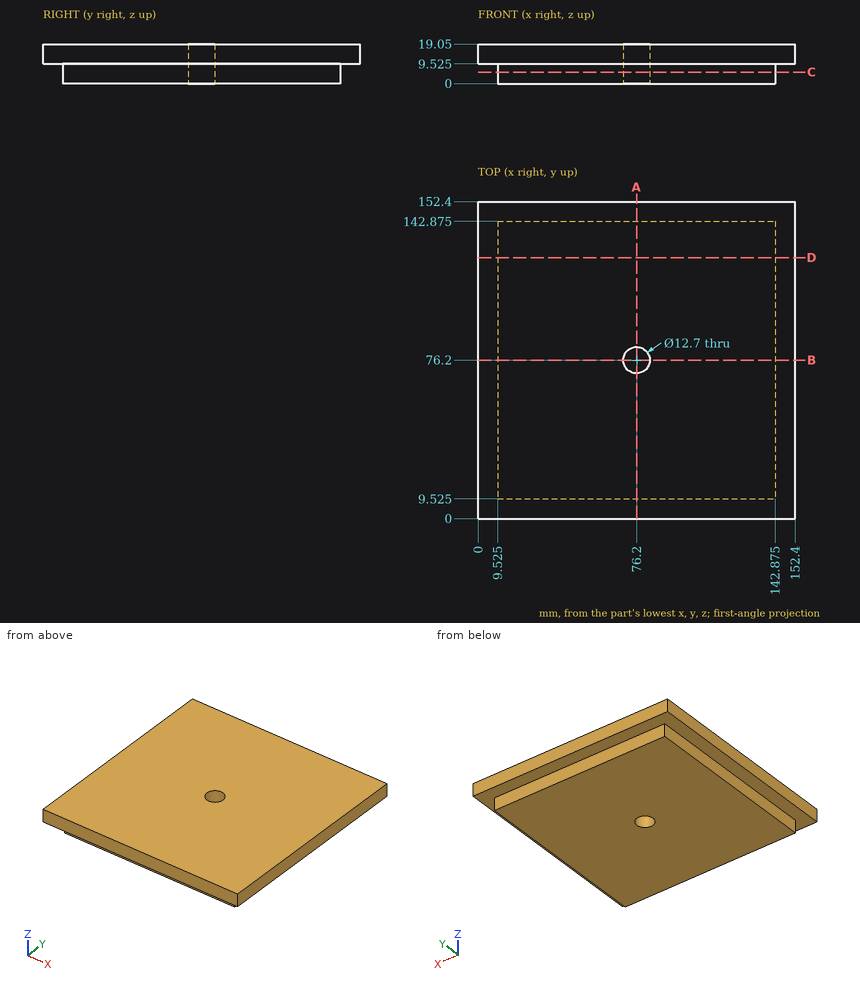
Design review of the part shown in the three views and the two pictorial views. Dimensions are in mm from the part's minimum x, y and z. Round coordinates to 2 decimals unless told otherwise and drop trailing zeros. Loops run counter-clockwise (first coordinate to the right, second up) from the corner with the lowest first, then second, coordinate; pieces in that order, holes last. Notation, with made-up numbers: M -1.75,-0.5 L 43.25,-0.5 A4 ccw 43.25,6.5 Z; hole C 8,50 d10. An arc over 180 degrees is marked long. Write item = value, one per line.
Item 1: Take a section at C-C on z = 5.5. Write out the cut boundary in (x, y) (3 decimals).
Return value:
outline = M 9.525,9.525 L 142.875,9.525 L 142.875,142.875 L 9.525,142.875 Z; hole C 76.2,76.2 d12.7
Item 2: Take a section at D-D on y = 125.5. Write out the cut boundary in (x, z) (3 decimals), then the cut area to 3 significant figures.
Return value:
outline = M 0,9.525 L 9.525,9.525 L 9.525,0 L 142.875,0 L 142.875,9.525 L 152.4,9.525 L 152.4,19.05 L 0,19.05 Z
area = 2,720 mm2
Item 3: Insertion check: P1, Ø3, axis at x = 84, z = 6.5, coming from the +Y side (3 decimals); P2, Ø4, axis at y = 78, z = 5, coming from the -X side (3 decimals); P3, Ø1, axis at x = 91.5, z = 4.5, coming from the -Y side (3 decimals). Each pin has a flat end and moves straight along its axis. Give the tip position at first contact, or say it passes through.
Return value:
P1 = 142.875
P2 = 9.525
P3 = 9.525
Item 4: Take a section at A-A on x = 76.2. Write out the cut boundary in (y, z) (3 decimals).
Return value:
outline = M 0,9.525 L 9.525,9.525 L 9.525,0 L 69.85,0 L 69.85,19.05 L 0,19.05 Z; M 82.55,0 L 142.875,0 L 142.875,9.525 L 152.4,9.525 L 152.4,19.05 L 82.55,19.05 Z
Item 5: For line 1 (Y direction, x = 76.2, z = 11.5); line 2 (Y direction, x = 76.2, z = 9.25) (3 decimals); line 3 (Y direction, x = 118.5, z = 6.25) (3 decimals), list the stretches that pass through material, from the lowest coordinate up. Write a range as [from, to].
Return value:
line_1 = [0, 69.85], [82.55, 152.4]
line_2 = [9.525, 69.85], [82.55, 142.875]
line_3 = [9.525, 142.875]
